Study the drawing (mm; zero at the part's minimum x, y, z) and answer. Coordinates: 2 decimals unless noted, no trailing zeros. Loops run counter-clockwise (first coordinate to the right, second up) from the corner with the lowest first, then second, coordinate; pieces in that order, holes last. Notation, with made-up numbers: (0, 19) - (32, 19) arc R10 ccw to (32, 36) - close; hole circle Ø10 at (27, 50.25). An arc over 180 degrees is marked (long way). Use one line per item in the form item = value.
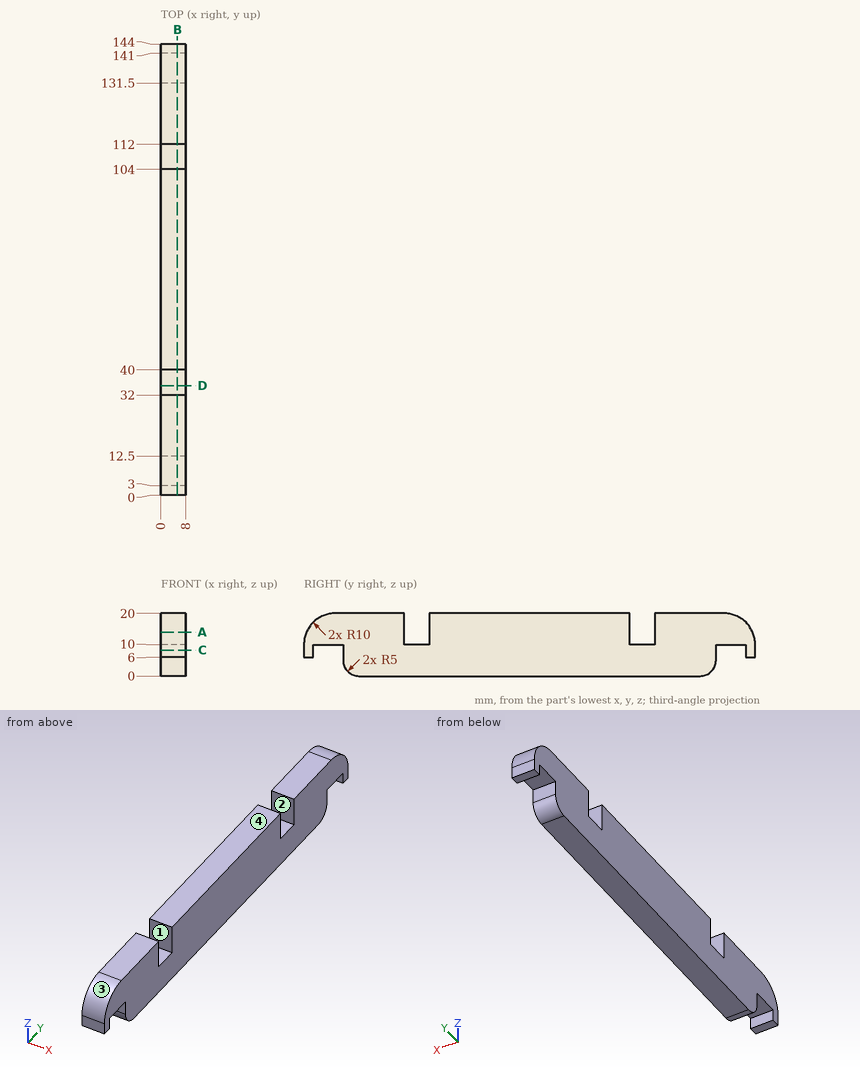
Item 1: The part is cut by section C-C on z = 8.25. Give the vertices of the cut face in (x, y), plus the area to 3 significant figures.
Results below:
outline = (0, 0) - (8, 0) - (8, 3) - (0, 3) - close; (0, 12.5) - (8, 12.5) - (8, 131.5) - (0, 131.5) - close; (0, 141) - (8, 141) - (8, 144) - (0, 144) - close
area = 1,000 mm²
Item 2: The part is cut by section A-A on z = 14. Give the vertices of the cut face in (x, y).
Results below:
outline = (0, 0.83) - (8, 0.83) - (8, 32) - (0, 32) - close; (0, 40) - (8, 40) - (8, 104) - (0, 104) - close; (0, 112) - (8, 112) - (8, 143.17) - (0, 143.17) - close
Item 3: The part is cut by section D-D on y = 35. Give the vertices of the cut face in (x, z).
Results below:
outline = (0, 0) - (8, 0) - (8, 10) - (0, 10) - close
Item 4: For a pull along Y with two mould halves and no side action, classify the marked faces 1, 2, 3 and 4 as +Y half, -Y half, draft (parallel to the pull), parting line (faces both ways), or undercut.
Results below:
face_1 = undercut
face_2 = undercut
face_3 = -Y half
face_4 = draft
Item 5: Find the intervals of material crossed by L1, parallel to Y at x = 5, z = 10.75; L2, parallel to Y at x = 6, z = 11.5; L3, parallel to Z at x = 3.25, y = 33, in increasing order.
Results below:
L1 = 0.03 to 32, 40 to 104, 112 to 143.97
L2 = 0.11 to 32, 40 to 104, 112 to 143.89
L3 = 0 to 10
Item 6: Each of these flat-tipped pins is pushed along its axis until it touches: P1, Ø2.5, axis at x = 2.5, y = 138.5, coming from the -Z side; P2, Ø0.9, axis at x = 3.5, y = 1.5, coming from the -Z side; P3, Ø4, axis at x = 5.5, z = 16.5, coming from the +Y side. Where does it stop, or does it pass through?
Results below:
P1 = 10
P2 = 6
P3 = 142.93
Item 7: The part is cut by section B-B on x = 5.25. Give the vertices of the cut face in (y, z).
Results below:
outline = (0, 6) - (3, 6) - (3, 10) - (12.5, 10) - (12.5, 5) arc R5 ccw to (17.5, 0) - (126.5, 0) arc R5 ccw to (131.5, 5) - (131.5, 10) - (141, 10) - (141, 6) - (144, 6) - (144, 10) arc R10 ccw to (134, 20) - (112, 20) - (112, 10) - (104, 10) - (104, 20) - (40, 20) - (40, 10) - (32, 10) - (32, 20) - (10, 20) arc R10 ccw to (0, 10) - close
